The model under review builds one solid part; all positions refer to its coordinate system, in mm. Face numbers are marked on the shaded views. A direction names the side the tool comes from. Coordinates: 2 decimals unless noted, no trailing zeros. Write each loop counter-clockwise with the first axis right and the second up, starting at its lowest first coordinate (ties: lowest second). Pieces come first, ordered by that corner, then holes. Notation, with made-up numbers: (69.5, 53) - (123.5, 53) arc R30 ccw to (123.5, 75) - close; hole circle Ø3 at (-25, 20). An arc over 180 degrees is marked (long way). Put each result on its own line as item: value.
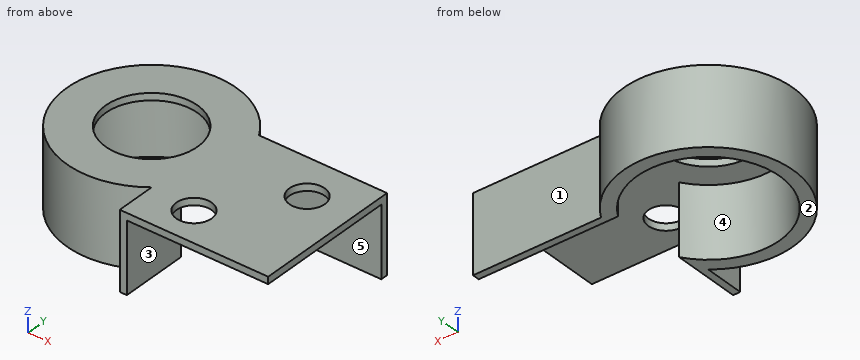
from build123d import *

# Parameters (mm, degrees)
CYLINDER041_R          = 6.5
CYLINDER041_DEPTH      = 11
CYLINDER030_R          = 2.5
CYLINDER030_DEPTH      = 11
CYLINDER031_R          = 2.5
CYLINDER031_DEPTH      = 11
BOX008_W               = 1
BOX008_H               = 7
BOX008_DEPTH           = 11
BOX010_W               = 20
BOX010_H               = 20
BOX010_DEPTH           = 1
CYLINDER035_R          = 12
CYLINDER035_DEPTH      = 1
PAD015_DEPTH           = 10
BOX011_W               = 177
BOX011_H               = 100
BOX011_DEPTH           = 10
CYLINDER029_R          = 7.5
CYLINDER029_DEPTH      = 10
CYLINDER038_R          = 10
CYLINDER038_DEPTH      = 10
CYLINDER039_R          = 7.5
CYLINDER039_DEPTH      = 10
CYLINDER032_R          = 10
CYLINDER032_DEPTH      = 10
PAD012_DEPTH           = 6.5
PAD013_DEPTH           = 4
PAD014_DEPTH           = 10
CYLINDER034_R          = 7.5
CYLINDER034_DEPTH      = 10
CYLINDER037_R          = 10
CYLINDER037_DEPTH      = 10
CYLINDER036_R          = 7.5
CYLINDER036_DEPTH      = 10
CYLINDER033_R          = 10
CYLINDER033_DEPTH      = 10
TUBE001_R              = 12
TUBE001_R_2            = 10.1
TUBE001_DEPTH          = 10
BOX009_W               = 19
BOX009_H               = 1
BOX009_DEPTH           = 11
CUT032_PLACEMENT_ANGLE = 180


with BuildPart() as cilindro041:
    # Cylinder041 → Cylinder041 (new body)
    with BuildSketch(Plane(origin=(97, 90, 0), x_dir=(1, 0, 0), z_dir=(0, 0, 1))):
        Circle(CYLINDER041_R)
    extrude(amount=CYLINDER041_DEPTH)


with BuildPart() as cilindro030:
    # Cylinder030 → Cylinder030 (new body)
    with BuildSketch(Plane(origin=(-83, 10, 0), x_dir=(1, 0, 0), z_dir=(0, 0, 1))):
        Circle(CYLINDER030_R)
    extrude(amount=CYLINDER030_DEPTH)


with BuildPart() as cilindro031:
    # Cylinder031 → Cylinder031 (new body)
    with BuildSketch(Plane(origin=(-75, 0, 0), x_dir=(1, 0, 0), z_dir=(0, 0, 1))):
        Circle(CYLINDER031_R)
    extrude(amount=CYLINDER031_DEPTH)


with BuildPart() as cubo004:
    # Box008 → Box008 (new body)
    with BuildSketch(Plane(origin=(-89.5, 8, 0), x_dir=(1, 0, 0), z_dir=(0, 0, 1))):
        with Locations((0.5, 3.5)):
            Rectangle(BOX008_W, BOX008_H)
    extrude(amount=BOX008_DEPTH)


with BuildPart() as cubo006:
    # Box010 → Box010 (new body)
    with BuildSketch(Plane(origin=(-88.5, -5, 10), x_dir=(1, 0, 0), z_dir=(0, 0, 1))):
        with Locations((10, 10)):
            Rectangle(BOX010_W, BOX010_H)
    extrude(amount=BOX010_DEPTH)


with BuildPart() as cilindro035:
    # Cylinder035 → Cylinder035 (new body)
    with BuildSketch(Plane(origin=(-97, 0, 10), x_dir=(1, 0, 0), z_dir=(0, 0, 1))):
        Circle(CYLINDER035_R)
    extrude(amount=CYLINDER035_DEPTH)


with BuildPart() as body011:
    # Sketch013 → Pad015 (new body)
    with BuildSketch(Plane.XY):
        Polygon((8.5, 4.907477), (0, 9.814955), (-8.5, 4.907477), (-8.5, -4.907477), (0, -9.814955), (8.5, -4.907477), align=None)
    extrude(amount=PAD015_DEPTH)


with BuildPart() as body011_1:
    # Body011 placement: moved
    add(body011.part.moved(Location((0, 45.1, 0))))


with BuildPart() as cut026:
    # Box011 → Box011 (new body)
    with BuildSketch(Plane(origin=(-88.5, -5, 0), x_dir=(1, 0, 0), z_dir=(0, 0, 1))):
        with Locations((88.5, 50)):
            Rectangle(BOX011_W, BOX011_H)
    extrude(amount=BOX011_DEPTH)

    # Cut026: cut Body011
    add(body011_1.part, mode=Mode.SUBTRACT)


with BuildPart() as cilindro029:
    # Cylinder029 → Cylinder029 (new body)
    with BuildSketch(Plane(origin=(0, 20, 0), x_dir=(1, 0, 0), z_dir=(0, 0, 1))):
        Circle(CYLINDER029_R)
    extrude(amount=CYLINDER029_DEPTH)


with BuildPart() as obj1:
    # Cylinder038 → Cylinder038 (new body)
    with BuildSketch(Plane(origin=(0, 20, 0), x_dir=(1, 0, 0), z_dir=(0, 0, 1))):
        Circle(CYLINDER038_R)
    extrude(amount=CYLINDER038_DEPTH)

    # Cut028: cut Cilindro029
    add(cilindro029.part, mode=Mode.SUBTRACT)


with BuildPart() as obj1_1:
    # Cut028 placement: moved
    add(obj1.part.moved(Location((-97, -20, 0))))


with BuildPart() as cilindro039:
    # Cylinder039 → Cylinder039 (new body)
    with BuildSketch(Plane(origin=(0, 20, 0), x_dir=(1, 0, 0), z_dir=(0, 0, 1))):
        Circle(CYLINDER039_R)
    extrude(amount=CYLINDER039_DEPTH)


with BuildPart() as fusion014:
    # Cylinder032 → Cylinder032 (new body)
    with BuildSketch(Plane(origin=(0, 20, 0), x_dir=(1, 0, 0), z_dir=(0, 0, 1))):
        Circle(CYLINDER032_R)
    extrude(amount=CYLINDER032_DEPTH)

    # Cut027: cut Cilindro039
    add(cilindro039.part, mode=Mode.SUBTRACT)


with BuildPart() as fusion014_1:
    # Cut027 placement: moved
    add(fusion014.part.moved(Location((97, -20, 0))))

    # Fusion014: union obj1
    add(obj1_1.part)


with BuildPart() as cuerpo006:
    # Sketch014 → Pad012 (new body)
    with BuildSketch(Plane.XY):
        Polygon((0, 7.505553), (-6.5, 3.752777), (-6.5, -3.752777), (0, -7.505553), (6.5, -3.752777), (6.5, 3.752777), align=None)
    extrude(amount=PAD012_DEPTH)

    # Sketch015 (on Face8 of Pad012) → Pad013 (join)
    with BuildSketch(Plane.XY.offset(6.5)):
        Polygon((0, 5.773503), (-5, 2.886751), (-5, -2.886751), (0, -5.773503), (5, -2.886751), (5, 2.886751), align=None)
    extrude(amount=PAD013_DEPTH)


with BuildPart() as cut029:
    # Sketch012 → Pad014 (new body)
    with BuildSketch(Plane.XY):
        Polygon((0, 9.814955), (-8.5, 4.907477), (-8.5, -4.907477), (0, -9.814955), (8.5, -4.907477), (8.5, 4.907477), align=None)
    extrude(amount=PAD014_DEPTH)

    # Cut029: cut Cuerpo006
    add(cuerpo006.part, mode=Mode.SUBTRACT)


with BuildPart() as cut029_1:
    # Cut029 placement: moved
    add(cut029.part.moved(Location((0, 45.1, 0))))


with BuildPart() as cilindro034:
    # Cylinder034 → Cylinder034 (new body)
    with BuildSketch(Plane(origin=(0, 20, 0), x_dir=(1, 0, 0), z_dir=(0, 0, 1))):
        Circle(CYLINDER034_R)
    extrude(amount=CYLINDER034_DEPTH)


with BuildPart() as obj2:
    # Cylinder037 → Cylinder037 (new body)
    with BuildSketch(Plane(origin=(0, 20, 0), x_dir=(1, 0, 0), z_dir=(0, 0, 1))):
        Circle(CYLINDER037_R)
    extrude(amount=CYLINDER037_DEPTH)

    # Cut030: cut Cilindro034
    add(cilindro034.part, mode=Mode.SUBTRACT)


with BuildPart() as obj2_1:
    # Cut030 placement: moved
    add(obj2.part.moved(Location((-97, -20, 0))))


with BuildPart() as cilindro036:
    # Cylinder036 → Cylinder036 (new body)
    with BuildSketch(Plane(origin=(0, 20, 0), x_dir=(1, 0, 0), z_dir=(0, 0, 1))):
        Circle(CYLINDER036_R)
    extrude(amount=CYLINDER036_DEPTH)


with BuildPart() as fusion011:
    # Cylinder033 → Cylinder033 (new body)
    with BuildSketch(Plane(origin=(0, 20, 0), x_dir=(1, 0, 0), z_dir=(0, 0, 1))):
        Circle(CYLINDER033_R)
    extrude(amount=CYLINDER033_DEPTH)

    # Cut033: cut Cilindro036
    add(cilindro036.part, mode=Mode.SUBTRACT)


with BuildPart() as fusion011_1:
    # Cut033 placement: moved
    add(fusion011.part.moved(Location((97, -20, 0))))

    # Fusion013: union obj2
    add(obj2_1.part)


with BuildPart() as fusion011_2:
    # Fusion013 placement: moved
    add(fusion011_1.part.moved(Location((0, 90, 0))))

    # Fusion011: union Cut026, Fusion014, Cut029
    add(cut026.part)
    add(fusion014_1.part)
    add(cut029_1.part)


with BuildPart() as cut031:
    # Tube001 → Tube001 (new body)
    with BuildSketch(Plane(origin=(-97, 0, 0), x_dir=(1, 0, 0), z_dir=(0, 0, 1))):
        Circle(TUBE001_R)
        Circle(TUBE001_R_2, mode=Mode.SUBTRACT)
    extrude(amount=TUBE001_DEPTH)

    # Cut031: cut Fusion011
    add(fusion011_2.part, mode=Mode.SUBTRACT)


with BuildPart() as obj3:
    # Box009 → Box009 (new body)
    with BuildSketch(Plane(origin=(-87.5, -6, 0), x_dir=(1, 0, 0), z_dir=(0, 0, 1))):
        with Locations((9.5, 0.5)):
            Rectangle(BOX009_W, BOX009_H)
    extrude(amount=BOX009_DEPTH)

    # Fusion012: union Cubo004, Cubo006, Cilindro035, Cut031
    add(cubo004.part)
    add(cubo006.part)
    add(cilindro035.part)
    add(cut031.part)

    # Cut025: cut Cilindro031
    add(cilindro031.part, mode=Mode.SUBTRACT)

    # Cut032: cut Cilindro030
    add(cilindro030.part, mode=Mode.SUBTRACT)


with BuildPart() as obj3_1:
    # Cut032 placement: moved
    add(obj3.part.moved(Location((0, 90, 0))).rotate(Axis((0, 90, 0), (0, 0, 1)), CUT032_PLACEMENT_ANGLE))

    # Cut035: cut Cilindro041
    add(cilindro041.part, mode=Mode.SUBTRACT)


with BuildPart() as eng_arandela_par:
    # Part__Mirroring001: instance of obj3
    add(obj3_1.part.mirror(Plane(origin=(0, 0, 0), x_dir=(0, -1, 0), z_dir=(1, 0, 0))))


solid = eng_arandela_par.part
1. Consider section B-B on y = 90. State the section outline as (x, z) points, plus the area to 3 significant figures.
Determined:
outline: (-109, 0) - (-107.1, 0) - (-107.1, 10) - (-103.5, 10) - (-103.5, 11) - (-109, 11) - close; (-90.5, 10) - (-77.5, 10) - (-77.5, 11) - (-90.5, 11) - close; (-72.5, 10) - (-68.5, 10) - (-68.5, 11) - (-72.5, 11) - close
area: 41.5 mm^2
2. For pin 1 Ø5 at (x, z) = (-74, 3.5) entering from -Y; pin 2 Ø4 at (x, y) = (-83, 80) entering from -Z; pin 3 Ø3 at (y, z) = (78.5, 4) entering from +X; pin 4 Ø5 at (x, z) = (-87.5, 6.5) entering from +Y, all flat-tipped, find the tip position at first contact; note any pin that passes through.
Determined:
pin 1: stops at y = 95
pin 2: passes through
pin 3: stops at x = -88.5
pin 4: stops at y = 99.75
3. Consider section C-C on z = 5. State the section outline as (x, y) points.
Determined:
outline: (-89.5, 75) - (-88.5, 75) - (-88.5, 84.54) arc R10.1 cw (long way) to (-88.22, 95) - (-68.5, 95) - (-68.5, 96) - (-86.61, 96) arc R12 ccw (long way) to (-89.5, 80.63) - close
4. The part is to be moulded in two halves that separate along Y. For the marked faces 3, 4 and 5, say which applies: +Y half, -Y half, draft (parallel to the pull), parting line (faces both ways), or undercut.
Determined:
face 3: draft
face 4: undercut
face 5: -Y half
5. Machinability: for the marked faces 1 and 2, which of the approach directions +Z, -Z, +X, -X, +Y, -Y give a long, thin tool a straight path to every point of the face, cutting with its end or side? Answer none if there is none.
Determined:
face 1: +Z, -Z, +X, +Y
face 2: -Z, +X, -X, +Y, -Y
6. Consider section A-A on x = -97. State the section outline as (y, z) points.
Determined:
outline: (78, 0) - (79.9, 0) - (79.9, 10) - (83.5, 10) - (83.5, 11) - (78, 11) - close; (96.5, 10) - (100.1, 10) - (100.1, 0) - (102, 0) - (102, 11) - (96.5, 11) - close
7. Consider section D-D on x = -81.5. State the section outline as (y, z) points.
Determined:
outline: (75, 10) - (78, 10) - (78, 11) - (75, 11) - close; (82, 10) - (95, 10) - (95, 0) - (96, 0) - (96, 11) - (82, 11) - close
8. To check wall thickness, follow probe 1 along Y at (x, z) = (-75, 10.75); probe 2 along Y at (x, z) = (-97, 4); probe 3 along X at (y, z) = (90, 10.35). State the ranges of each line that lie inside material, in increasing order.
Determined:
probe 1: y = 75 to 87.5, 92.5 to 96
probe 2: y = 78 to 79.9, 100.1 to 102
probe 3: x = -109 to -103.5, -90.5 to -77.5, -72.5 to -68.5
